```python
from build123d import *

# Parameters (mm, degrees)
BOSS_EXTRUDE2_DEPTH = 24.3
SKETCH5_R           = 3
CUT_EXTRUDE1_DEPTH  = 10
SKETCH10_R          = 3
CUT_EXTRUDE2_DEPTH  = 10


with BuildPart() as part:
    # Sketch4 → Boss-Extrude2 (new, symmetric)
    with BuildSketch(Plane.ZY.offset(-117.5682)):
        Polygon((-1089.668968128, 78.04), (-1089.668968128, 264.04), (-855.402894198, 532.098588009), (-742.813619106, 508.675199397), (-846.747853315, 78.04), (-849.333608688, 78.664074634), (-746.043555874, 506.630209448), (-854.422864001, 529.177744724), (-1087.008968128, 263.041459529), (-1087.008968128, 78.04), align=None)
    extrude(amount=BOSS_EXTRUDE2_DEPTH, both=True)

    # Sketch5 → Cut-Extrude1 (cut)
    with BuildSketch(Plane(origin=(0, 0, -1089.668968128), x_dir=(-1, 0, 0), z_dir=(0, 0, -1))):
        with Locations((-117.5682, 90.04090214)):
            Circle(SKETCH5_R)
    extrude(amount=-CUT_EXTRUDE1_DEPTH, mode=Mode.SUBTRACT)

    # Sketch10 → Cut-Extrude2 (cut)
    with BuildSketch(Plane(origin=(0, 198.034168105, -820.523517758), x_dir=(-1, 0, 0), z_dir=(0, 0.23461452417479184, -0.9720884862224406))):
        with Locations(Location((-117.5682, -111.819624777, 0), (0, 0, 90))):
            Circle(SKETCH10_R)
    extrude(amount=-CUT_EXTRUDE2_DEPTH, mode=Mode.SUBTRACT)


solid = part.part
```
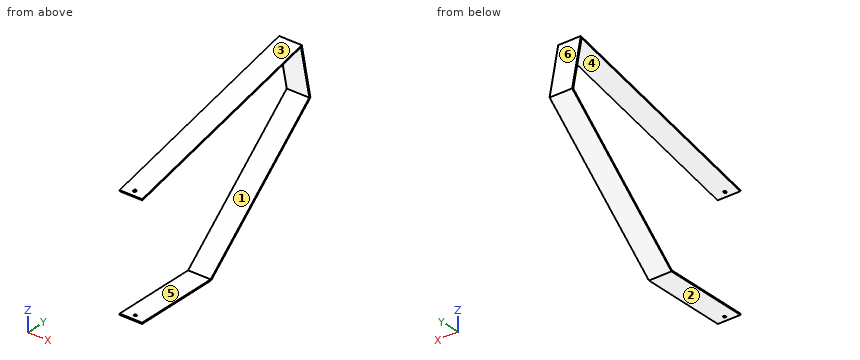
The listing builds one solid part. Answer for the finished solid, in the listing's coordinates (mm). Face numbers are marked on the shaded views. A direction names the side the tool comes from. Give positions to 0.01 mm unless a question says otherwise; leave off trailing zeros. Order: outer loops, then holes, each group sorted by start corner. A loop starts at its lowest first (then second) coordinate and runs counter-clockwise, first axis right, second up.
Item 1: The part is cut by section D-D, the plane z = -895. Give the vertices of the cut face in (x, y).
From the geometry:
outline: (93.27, 482.75) - (141.87, 482.75) - (141.87, 486.79) - (93.27, 486.79) - close
Item 2: Which of the six approach directions +Z, -Z, +X, -X, +Y, -Y give full straight-line access (tool end or side, diameter ignored) to the marked faces 4, 5 and 6?
From the geometry:
face 4: +X, -X
face 5: +X, -X, -Y
face 6: +Z, +X, -X, +Y
Item 3: Find the intervals of material crossed by probe 1 along Z at (x, y) = (118.5, 98); probe 2 along Z at (x, y) = (133.5, 113); probe 3 along Y at (x, z) = (114, -869.5), in increasing order.
From the geometry:
probe 1: z = -1089.67 to -1087.01, -844.67 to -841.93
probe 2: z = -1089.67 to -1087.01, -841.05 to -838.31
probe 3: y = 511.93 to 515.97
Item 4: The part is cut by section A-A, the plane x = 136. Give the vertices of the cut face in (y, z).
From the geometry:
outline: (78.04, -1089.67) - (264.04, -1089.67) - (532.1, -855.4) - (508.68, -742.81) - (78.04, -846.75) - (78.66, -849.33) - (506.63, -746.04) - (529.18, -854.42) - (263.04, -1087.01) - (78.04, -1087.01) - close
Item 5: Given pin 1 Ø5 at (x, z) = (99, -872.5) entering from +Y; pin 2 Ø10 at (x, z) = (99, -809) entering from +Y (3 decimals); pin 3 Ø8 at (x, y) = (117.57, 90.04) entering from +Z, each flat-ended and moving along its own axis, determine where each tip first touches the part or whether it passes through.
From the geometry:
pin 1: stops at y = 515.4
pin 2: stops at y = 523.485
pin 3: stops at z = -842.89
Item 6: The part is cut by section B-B, the plane y = 271. Give the vertices of the cut face in (x, z), and give its area (3 significant figures).
From the geometry:
outline: (93.27, -1083.59) - (141.87, -1083.59) - (141.87, -1080.05) - (93.27, -1080.05) - close; (93.27, -802.91) - (141.87, -802.91) - (141.87, -800.18) - (93.27, -800.18) - close
area: 305 mm2
Item 7: For a pull along Z with two mould halves and no side action, classify the marked faces 1, 2 and 3 as pulls with the +Z half, pulls with the -Z half, needs draft (parallel to the pull), parting line crosses it, or undercut.
From the geometry:
face 1: undercut
face 2: pulls with the -Z half
face 3: pulls with the +Z half
Item 8: The part is cut by section C-C, the plane z = -804. Give the vertices of the cut face in (x, y).
From the geometry:
outline: (93.27, 255.16) - (141.87, 255.16) - (141.87, 266.5) - (93.27, 266.5) - close; (93.27, 518.69) - (141.87, 518.69) - (141.87, 521.4) - (93.27, 521.4) - close
